For this review, take the finished solid that the model builds, in its own axes (mm). Coordinates: 2 decimals unless noted, no trailing zeros. Loops run counter-clockwise (first coordinate to the right, second up) from the corner with the lowest first, then second, coordinate; pieces in that order, holes last. Notation, with made-up numbers: (0, 12.5) -> (27, 12.5) arc R29 cw to (27, 32.5) -> close; hole circle Ø3 at (13.5, 79.5). An arc over 180 degrees is marked (long way). Answer in a Markdown table with one row per item.
from build123d import *

# Parameters (mm, degrees)
F0_W     = 114.3
F0_H     = 127
F1_DEPTH = 0.8636
F3_DEPTH = 0.8636
F4_R     = 5.08
F6_D     = 3.7973
F8_D     = 3.7973


with BuildPart() as f1:
    # F0 (on Front) → F1 (new body)
    with BuildSketch(Plane.XZ):
        Rectangle(F0_W, F0_H)
    extrude(amount=-F1_DEPTH)

    # F2 (on face) → F3 (cut, through all)
    with BuildSketch(Plane.XZ):
        with BuildLine():
            ThreePointArc((-16.0869264489, 35.5412906039), (-16.5518944338, 36.663822619), (-17.6744264489, 37.1287906039))
            Line((-17.6744264489, 37.1287906039), (-41.8044264489, 37.1287906039))
            ThreePointArc((-41.8044264489, 37.1287906039), (-42.9269584641, 36.663822619), (-43.3919264489, 35.5412906039))
            Line((-43.3919264489, 35.5412906039), (-43.3919264489, 18.7518906039))
            ThreePointArc((-43.3919264489, 18.7518906039), (-42.9269584641, 17.6293585888), (-41.8044264489, 17.1643906039))
            Line((-41.8044264489, 17.1643906039), (-17.6744264489, 17.1643906039))
            ThreePointArc((-17.6744264489, 17.1643906039), (-16.5518944338, 17.6293585888), (-16.0869264489, 18.7518906039))
            Line((-16.0869264489, 18.7518906039), (-16.0869264489, 35.5412906039))
        make_face()
        with BuildLine():
            ThreePointArc((36.2763346143, 35.5412906039), (35.8113666294, 36.663822619), (34.6888346143, 37.1287906039))
            Line((34.6888346143, 37.1287906039), (5.2248346143, 37.1287906039))
            ThreePointArc((5.2248346143, 37.1287906039), (4.1023025991, 36.663822619), (3.6373346143, 35.5412906039))
            Line((3.6373346143, 35.5412906039), (3.6373346143, -27.7047093961))
            ThreePointArc((3.6373346143, -27.7047093961), (4.1023025991, -28.8272414112), (5.2248346143, -29.2922093961))
            Line((5.2248346143, -29.2922093961), (34.6888346143, -29.2922093961))
            ThreePointArc((34.6888346143, -29.2922093961), (35.8113666294, -28.8272414112), (36.2763346143, -27.7047093961))
            Line((36.2763346143, -27.7047093961), (36.2763346143, 35.5412906039))
        make_face()
    extrude(amount=-F3_DEPTH, mode=Mode.SUBTRACT)

    # F4
    f4_edges = [f1.edges().sort_by_distance(p)[0] for p in [
        (-57.15, 0.4318, 63.5),
        (57.15, 0.4318, 63.5),
        (57.15, 0.4318, -63.5),
        (-57.15, 0.4318, -63.5),
    ]]
    fillet(f4_edges, radius=F4_R)

    # F6 (through all)
    with Locations(Plane.XZ):
        with Locations((19.9568346143, 52.0639906039), (19.9568346143, -44.6846093961)):
            Hole(F6_D / 2)

    # F8 (through all)
    with Locations(Plane.XZ):
        with Locations((-50.8, 57.15), (50.8, 57.15), (50.8, -57.15), (-50.8, -57.15)):
            Hole(F8_D / 2)


solid = f1.part
Item 1: For L1, parallel to X at y = 0.8, z = 19.5; L2, parallel to Z at x = -50.8, y = 0.75; L3, parallel to X at y = 0.7, z = -5, list the stretches that pass through material, from the lowest coordinate up.
Worked answers:
| item | result |
|---|---|
| L1 | -57.15 to -43.39, -16.09 to 3.64, 36.28 to 57.15 |
| L2 | -63.5 to -59.05, -55.25 to 55.25, 59.05 to 63.5 |
| L3 | -57.15 to 3.64, 36.28 to 57.15 |
Item 2: Take a section at B-B, the plane y = 0.55. Count the separate pieces of the cut face and the enclosed holes in it, and give its area (3 significant figures).
Worked answers:
| item | result |
|---|---|
| separate pieces | 1 |
| enclosed holes | 8 |
| area | 11,700 mm² |
Item 3: The part is to be moulded in two halves that separate along Z. For faces 1 (the flat face through (-1, 0.864, 1)), 2 (the cylindrical face through (55.622, 0.438, 62.051)), 3 (the cylindrical face through (-55.701, 0.438, -61.972)), 4 (the cylindrical face through (20.2, 0.4, -42.8)), say which applies: +Z half, -Z half, draft (parallel to the pull), parting line (faces both ways), or undercut.
Worked answers:
| item | result |
|---|---|
| face 1 | draft |
| face 2 | +Z half |
| face 3 | -Z half |
| face 4 | undercut |
Item 4: Take a section at A-A, the plane z = 13.5. State the section outline as (x, y) points, and give its area (3 significant figures).
Worked answers:
| item | result |
|---|---|
| outline | (-57.15, 0) -> (3.64, 0) -> (3.64, 0.86) -> (-57.15, 0.86) -> close; (36.28, 0) -> (57.15, 0) -> (57.15, 0.86) -> (36.28, 0.86) -> close |
| area | 70.5 mm² |
